Read the model definition and answer for the solid it produces. Units are mm, in the model's axes. Face numbers are marked on the shaded views. A direction names the side the tool comes from. Coordinates: 2 decimals unless noted, no trailing zeros. Loops run counter-clockwise (first coordinate to the right, second up) from the corner with the lowest first, then second, coordinate; pieces in that order, holes last. Notation, with made-up numbers: (62, 70) -> (83, 70) arc R30 ccw to (83, 93) -> close; hole circle Ø1 at (35.25, -14). An arc over 180 degrees is marked (long way). Answer in a Markdown table with one row per item.
Autodesk Inventor part; units mm, degrees
ref_plane "YZ Plane" through (0, 0, 0) normal (1, 0, 0) x (0, 1, 0)
ref_plane "XZ Plane" through (0, 0, 0) normal (0, 1, 0) x (-1, 0, 0)
ref_plane "XY Plane" through (0, 0, 0) normal (0, 0, 1) x (1, 0, 0)
sketch "Sketch1" plane through (0, 0, 0) normal (0, 0, 1) x (1, 0, 0)
  line L0 (0, 0) -> (10, 0)
  line L1 (0, 0) -> (0, 5)
  line L2 (0, 5) -> (11.504, 5)
  arc A0 (11.504, 5) -> (21.3051, 5) centre (16.4046, 6.5) ccw
  arc A1 (10, 0) -> (22.8091, 0) centre (16.4046, 6.5) ccw
  line L3 (21.3051, 5) -> (32.8091, 5)
  line L4 (32.8091, 5) -> (32.8091, 0)
  line L5 (32.8091, 0) -> (22.8091, 0)
  dimension "d0" = 10
  dimension "d1" = 11.504
  dimension "d2" = 5
  dimension "d3" = 5.125
  dimension "d4" = 1.5
extrude "Extrusion1" add sketch "Sketch1" along normal blind 10
sketch "Sketch2" plane through (22.8091, 0, 0) normal (0, -1, 0) x (1, 0, 0)
  line L0 (0, 0) -> (10, 0)
  line L1 (10, 0) -> (10, 10)
  line L2 (0, 10) -> (10, 10)
  line L3 (0, 0) -> (0, 10)
  line L4 (-22.8091, 0) -> (-12.8091, 0)
  line L5 (-12.8091, 0) -> (-12.8091, 10)
  line L6 (-22.8091, 10) -> (-12.8091, 10)
  line L7 (-22.8091, 0) -> (-22.8091, 10)
  line L8 (-22.8091, 0) -> (-22.8091, 10)
  line L9 (-22.8091, 10) -> (-12.8091, 0)
  line L10 (-22.8091, 0) -> (-12.8091, 10)
  line L11 (0, 10) -> (10, 0)
  line L12 (0, 0) -> (10, 0)
  line L13 (0, 0) -> (10, 10)
  point P0 (-17.8091, 5)
  point P1 (5, 5)
hole "Hole1" at (5, 0, 5) at (27.8091, 0, 5) direction (0, 1, 0) diameter 4.305 end through all
properties part number "clampCap"
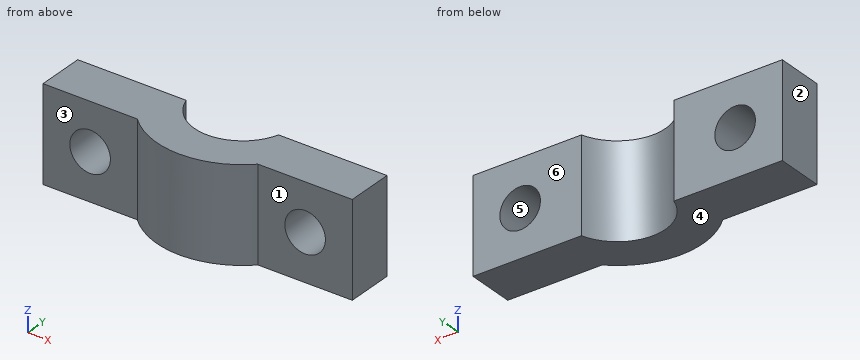
1. Find the intervals of material crossed by probe 1 along X at (y, z) = (1.2, 5); probe 2 along X at (y, z) = (3, 5); probe 3 along X at (y, z) = (2.75, 3.25), in increasing order.
A:
| item | result |
|---|---|
| probe 1 | x = 0 to 2.85, 7.15 to 25.66, 29.96 to 32.81 |
| probe 2 | x = 0 to 2.85, 7.15 to 12.66, 20.15 to 25.66, 29.96 to 32.81 |
| probe 3 | x = 0 to 3.75, 6.25 to 12.91, 19.9 to 26.56, 29.06 to 32.81 |
2. The mould has two halves that part along Z. Classify the marked faces 4, 5 and 6: pulls with the +Z half, pulls with the -Z half, needs draft (parallel to the pull), parting line crosses it, or undercut.
A:
| item | result |
|---|---|
| face 4 | pulls with the -Z half |
| face 5 | undercut |
| face 6 | needs draft |
3. A cutting plane is placed at D-D on z = 1. Give the vertices of the cut face in (x, y).
A:
| item | result |
|---|---|
| outline | (0, 0) -> (10, 0) arc R9.13 ccw to (22.81, 0) -> (32.81, 0) -> (32.81, 5) -> (21.31, 5) arc R5.12 cw to (11.5, 5) -> (0, 5) -> close |
4. A cutting plane is placed at A-A on z = 5. Give the vertices of the cut face in (x, y).
A:
| item | result |
|---|---|
| outline | (0, 0) -> (2.85, 0) -> (2.85, 5) -> (0, 5) -> close; (7.15, 0) -> (10, 0) arc R9.13 ccw to (22.81, 0) -> (25.66, 0) -> (25.66, 5) -> (21.31, 5) arc R5.12 cw to (11.5, 5) -> (7.15, 5) -> close; (29.96, 0) -> (32.81, 0) -> (32.81, 5) -> (29.96, 5) -> close |
5. A cutting plane is placed at C-C on x = 5. Give the vertices of the cut face in (y, z), and give its area (3 significant figures).
A:
| item | result |
|---|---|
| outline | (0, 0) -> (5, 0) -> (5, 2.85) -> (0, 2.85) -> close; (0, 7.15) -> (5, 7.15) -> (5, 10) -> (0, 10) -> close |
| area | 28.5 mm2 |
6. Given pin 1 Ø4 at (x, z) = (24, 9) entering from -Y; pin 2 Ø3 at (x, z) = (29.5, 7) entering from -Y, each flat-ended and moving along its own axis, determine where each tip first touches the part or whether it passes through.
A:
| item | result |
|---|---|
| pin 1 | stops at y = -0.71 |
| pin 2 | stops at y = 0 |
7. A tool of negligible diameter and unlimited length cuts with its end or side. For the marked faces 1, 2 and 3, from which of +Z, -Z, +X, -X, +Y, -Y can it reach the whole face along a straight path? Write none if from no direction.
A:
| item | result |
|---|---|
| face 1 | +Z, -Z, +X, -Y |
| face 2 | +Z, -Z, -X, +Y, -Y |
| face 3 | +Z, -Z, -X, -Y |
8. A cutting plane is placed at B-B on y = 2.75. Give the vertices of the cut face in (x, z) (1 decimal).
A:
| item | result |
|---|---|
| outline | (0, 0) -> (12.9, 0) -> (12.9, 10) -> (0, 10) -> close; (19.9, 0) -> (32.8, 0) -> (32.8, 10) -> (19.9, 10) -> close; hole circle Ø4.3 at (5, 5); hole circle Ø4.3 at (27.8, 5) |
